from build123d import *

# Parameters (mm, degrees)
SKETCH2_R          = 4.15
CUT_EXTRUDE1_DEPTH = 10
SKETCH3_R          = 1.4
CUT_EXTRUDE3_DEPTH = 30
CIRPATTERN1_COUNT  = 4
FILLET1_R          = 2
SKETCH4_R          = 1.6
CUT_EXTRUDE4_DEPTH = 19.0000001
SKETCH6_R          = 2.75
CUT_EXTRUDE5_DEPTH = 0.85


with BuildPart() as part:
    # Sketch1 → Revolve1 (revolve)
    with BuildSketch(Plane.XY):
        Polygon((0, 0), (0, 2), (23, 2), (23, 18), (25, 18), (25, 0), align=None)
    revolve(axis=Axis((0, 0, 0), (0, 1, 0)))

    # Sketch2 → Cut-Extrude1 (cut)
    with BuildSketch(Plane(origin=(0, 2, 0), x_dir=(1, 0, 0), z_dir=(0, 1, 0))):
        Circle(SKETCH2_R)
    extrude(amount=-CUT_EXTRUDE1_DEPTH, mode=Mode.SUBTRACT)

    # Sketch3 → Cut-Extrude3 (cut, symmetric)
    with BuildSketch(Plane.XY):
        with Locations((0, 9)):
            Circle(SKETCH3_R)
    cut_extrude3 = extrude(amount=CUT_EXTRUDE3_DEPTH, both=True, mode=Mode.SUBTRACT)

    # CirPattern1: Cut-Extrude3 ×4 about axis
    cirpattern1_axis = Axis((0, 0, 0), (0, -1, 0))
    for i in range(1, CIRPATTERN1_COUNT):
        add(cut_extrude3.rotate(cirpattern1_axis, i * 360 / CIRPATTERN1_COUNT), mode=Mode.SUBTRACT)

    # Fillet1
    fillet1_edges = [part.edges().sort_by_distance(p)[0] for p in [
        (-25, 0, 0),
    ]]
    fillet(fillet1_edges, radius=FILLET1_R)

    # Sketch4 → Cut-Extrude4 (cut, through all)
    with BuildSketch(Plane.XZ):
        with Locations((-3.5, 8)):
            Circle(SKETCH4_R)
        with Locations((3.5, 8)):
            Circle(SKETCH4_R)
        with Locations((-8, 3.5)):
            Circle(SKETCH4_R)
        with Locations((8, 3.5)):
            Circle(SKETCH4_R)
    cut_extrude4 = extrude(amount=-CUT_EXTRUDE4_DEPTH, mode=Mode.SUBTRACT)

    # Sketch6 → Cut-Extrude5 (cut)
    with BuildSketch(Plane(origin=(0, 2, 0), x_dir=(1, 0, 0), z_dir=(0, 1, 0))):
        with Locations((-8, -3.5)):
            Circle(SKETCH6_R)
        with Locations((-3.5, -8)):
            Circle(SKETCH6_R)
        with Locations((3.5, -8)):
            Circle(SKETCH6_R)
        with Locations((8, -3.5)):
            Circle(SKETCH6_R)
    cut_extrude5 = extrude(amount=-CUT_EXTRUDE5_DEPTH, mode=Mode.SUBTRACT)

    # Mirror1: Cut-Extrude4, Cut-Extrude5 across plane
    add(cut_extrude4.mirror(Plane.XY), mode=Mode.SUBTRACT)
    add(cut_extrude5.mirror(Plane.XY), mode=Mode.SUBTRACT)


solid = part.part
CAD build for the part. Positions are in the model's coordinates, mm. A direction names the side the tool comes from. Round coordinates to 2 decimals unless told otherwise and drop trailing zeros. Order: outer loops, then holes, each group sorted by start corner. A loop starts at its lowest first (then second) coordinate and runs counter-clockwise, first axis right, second up. Notation, with made-up numbers: (28, 0) -> (80, 0) arc R10 cw to (80, 12) -> close; hole circle Ø8 at (17, 6.5). An arc over 180 degrees is marked (long way). Write item = value, one per line. Start each with the question number.
(1) Cut at D-D, the plane x = -8. State how many separate pieces and enclosed holes the cut face has, then the cut area to 3 significant figures.
(2) Cut at B-B, the plane y = 9. List the corners of the cut face in (x, z).
(3) Which spindle directions (+Z, -Z, +X, -X, +Y, -Y) get a long thin tool onto all of the face, cutting with end or side? Do faces 1 (the cylindrical face through (23.96, 10.18, 0.75)), 2 (the cylindrical face through (-6.73, 1.58, -5.94)). Say none if no direction does.
(4) Cut at C-C, the plane y = 4. List the corners of the cut face in (x, z).
(5) Pin check, flat tips, straight feed: P1, Ø1.5, axis at x = -9.5, z = 13.5, coming from the +Y side; P2, Ø1.5, axis at x = 3, y = 15.5, coming from the +Z side; P3, Ø1.6, axis at x = -4.5, z = -9, coming from the +Y side; P4, Ø8, axis at x = 6.5, z = 3, coming from the -Y side. Stop position of each tip, or through.
(6) Probe line 1 (Z direction, x = 8, y = 0.5); line 2 (Z direction, x = 0, y = 6.5); line 3 (Z direction, x = -3.5, y = 0.85). List the from-to ranges inside material, lowest first. Write a range as [from, to].
(7) Cut at A-A, the plane z = 0. List the corners of the cut face in (x, y).
(8) Pull direction Z, two halves, no side cores. Call faces 3 (the cylindrical face through (23.846, 9.888, -7.509)), 4 (the cylindrical face through (0.75, 10.18, -23.96)), 5 (the cylindrical face through (-9.6, 0.57, -3.57)): released by +Z, released by -Z, zero draft, split by the parting line, or undercut.
Model answer:
q1.separate_pieces = 3
q1.enclosed_holes = 0
q1.area = 144 mm2
q2.outline = (-24.96, -1.4) arc R25 ccw to (-1.4, -24.96) -> (-1.4, -22.96) arc R23 cw to (-22.96, -1.4) -> close; (-24.96, 1.4) -> (-22.96, 1.4) arc R23 cw to (-1.4, 22.96) -> (-1.4, 24.96) arc R25 ccw to start; (1.4, -24.96) arc R25 ccw to (24.96, -1.4) -> (22.96, -1.4) arc R23 cw to (1.4, -22.96) -> close; (1.4, 22.96) arc R23 cw to (22.96, 1.4) -> (24.96, 1.4) arc R25 ccw to (1.4, 24.96) -> close
q3.face_1 = +X, -X
q3.face_2 = +Y
q4.outline = circle Ø50 at (0, 0); hole circle Ø46 at (0, 0)
q5.P1 = 2
q5.P2 = 24.9
q5.P3 = 1.15
q5.P4 = 0
q6.line_1 = [-22.97, -5.1], [-1.9, 1.9], [5.1, 22.97]
q6.line_2 = [-25, -23], [23, 25]
q6.line_3 = [-24.39, -9.6], [-6.4, -2.23], [2.23, 6.4], [9.6, 24.39]
q7.outline = (-25, 2) arc R2 ccw to (-23, 0) -> (-4.15, 0) -> (-4.15, 2) -> (-23, 2) -> (-23, 7.6) -> (-25, 7.6) -> close; (-25, 10.4) -> (-23, 10.4) -> (-23, 18) -> (-25, 18) -> close; (4.15, 0) -> (23, 0) arc R2 ccw to (25, 2) -> (25, 7.6) -> (23, 7.6) -> (23, 2) -> (4.15, 2) -> close; (23, 10.4) -> (25, 10.4) -> (25, 18) -> (23, 18) -> close
q8.face_3 = split by the parting line
q8.face_4 = zero draft
q8.face_5 = undercut
